Can you work these out from the model? Positions are in its coordinate system, mm. Coordinates: 2 decimals unless noted, no trailing zeros. Loops run counter-clockwise (first coordinate to the right, second up) from the corner with the lowest first, then second, coordinate; pieces in that order, holes last. Notation, with made-up numbers: (-22.75, -13) -> (29.25, -13) arc R15 ccw to (29.25, 11) -> close; hole circle Ø3 at (-28, 21.5). An arc over 180 degrees is marked (long way). Put each result on its own line as item: value. Start each with the question number.
Item 1: Please list where these lines run through material, in increasing order: L1, parallel to Z at x = 0, y = 2.75; L2, parallel to Z at x = 0.5, y = 5.25; L3, parallel to X at y = 0, z = 260.35. Write a range as from..to.
Item 2: If we section it at A-A on z = -216: Please give me the cut outline in (x, y), plus the area to 3 significant figures.
Item 3: Will these pins go through, and if not, where does the flat tip stop? P1, Ø6, axis at y = 4, z = 188.5, coming from the +X side (3 decimals); P2, Ø5, axis at y = -0.5, z = 37, coming from the +X side.
Item 4: If we section it at B-B on y = -2.75: Please give me the cut outline in (x, z), plus the area to 3 significant figures.
```python
from build123d import *

# Parameters (mm, degrees)
BOSS_EXTRUDE1_DEPTH = 266.7
SKETCH2_R           = 1.2573
CUT_EXTRUDE1_DEPTH  = 13.7


with BuildPart() as part:
    # Sketch1 → Boss-Extrude1 (new body, symmetric)
    with BuildSketch(Plane.XY):
        Polygon((3.666174209, -6.35), (7.332348419, 0), (3.666174209, 6.35), (-3.666174209, 6.35), (-7.332348419, 0), (-3.666174209, -6.35), align=None)
    extrude(amount=BOSS_EXTRUDE1_DEPTH, both=True)

    # Sketch2 → Cut-Extrude1 (cut, through all)
    with BuildSketch(Plane(origin=(0, 6.35, 0), x_dir=(1, 0, 0), z_dir=(0, 1, 0))):
        with Locations((0, -260.35)):
            Circle(SKETCH2_R)
        with Locations((0, 260.35)):
            Circle(SKETCH2_R)
    extrude(amount=-CUT_EXTRUDE1_DEPTH, mode=Mode.SUBTRACT)


solid = part.part
```
Solutions:
1. L1: -266.7..-261.61, -259.09..259.09, 261.61..266.7
1. L2: -266.7..-261.5, -259.2..259.2, 261.5..266.7
1. L3: -7.33..-1.26, 1.26..7.33
2. outline: (-7.33, 0) -> (-3.67, -6.35) -> (3.67, -6.35) -> (7.33, 0) -> (3.67, 6.35) -> (-3.67, 6.35) -> close
2. area: 140 mm^2
3. P1: x = 6.755
3. P2: x = 7.33
4. outline: (-5.74, -266.7) -> (5.74, -266.7) -> (5.74, 266.7) -> (-5.74, 266.7) -> close; hole circle Ø2.51 at (0, -260.35); hole circle Ø2.51 at (0, 260.35)
4. area: 6,120 mm^2
